Verification items for this drawing (mm, ordinates from the low corner). A direction names the side the tool comes from. Round coordinates to 2 decimals unless told otherwise and drop trailing zeros. Order: outer loops, then holes, each group sorted by start corner. A loop starts at its lowest first (then second) coordinate and runs counter-clockwise, first axis right, second up. Notation, with made-up numbers: (-8.75, -14.5) -> (8.25, -14.5) arc R19 ccw to (8.25, -2.5) -> close; hole circle Ø11 at (29, -28.75). An arc over 180 degrees is marked (long way). Answer in a Markdown table with one row per item. Add a question column.
1. Sectioned sample at B-B, the plane y = 33. Record the boundary of the cut face in (x, z) (3 decimals).
2. Access from +Z, -Z, +X, -X, +Y, -Y to the whole of each face (thin tool, end or side, straight path). Record for the marked faces 4 and 5.
3. Material ranges on L1, parallel to Z at x = 155, y = 62; L2, parallel to X at y = 96.5, z = 453, recorded low to high. Write a range as from..to.
4. Depth check by flat-ended pin: P1, Ø10, axis at x = 90, y = 67.5, coming from the -Z side; P2, Ø10, axis at y = 71, z = 347.5, coming from the +X side. Enter the tip coordinate at first touch or a pass-through.
5. Draft check along Z on the marked faces 1, 2 and 3. Enter one of: +Z half, -Z half, draft (parallel to the pull), parting line (faces both ways), or undercut.
6. Sectioned sample at C-C, the plane z = 95.5. Record the boundary of the cut face in (x, y).
7. Sectioned sample at A-A, the plane x = 233. Record the boundary of the cut face in (y, z), then the cut area to 3 significant figures.
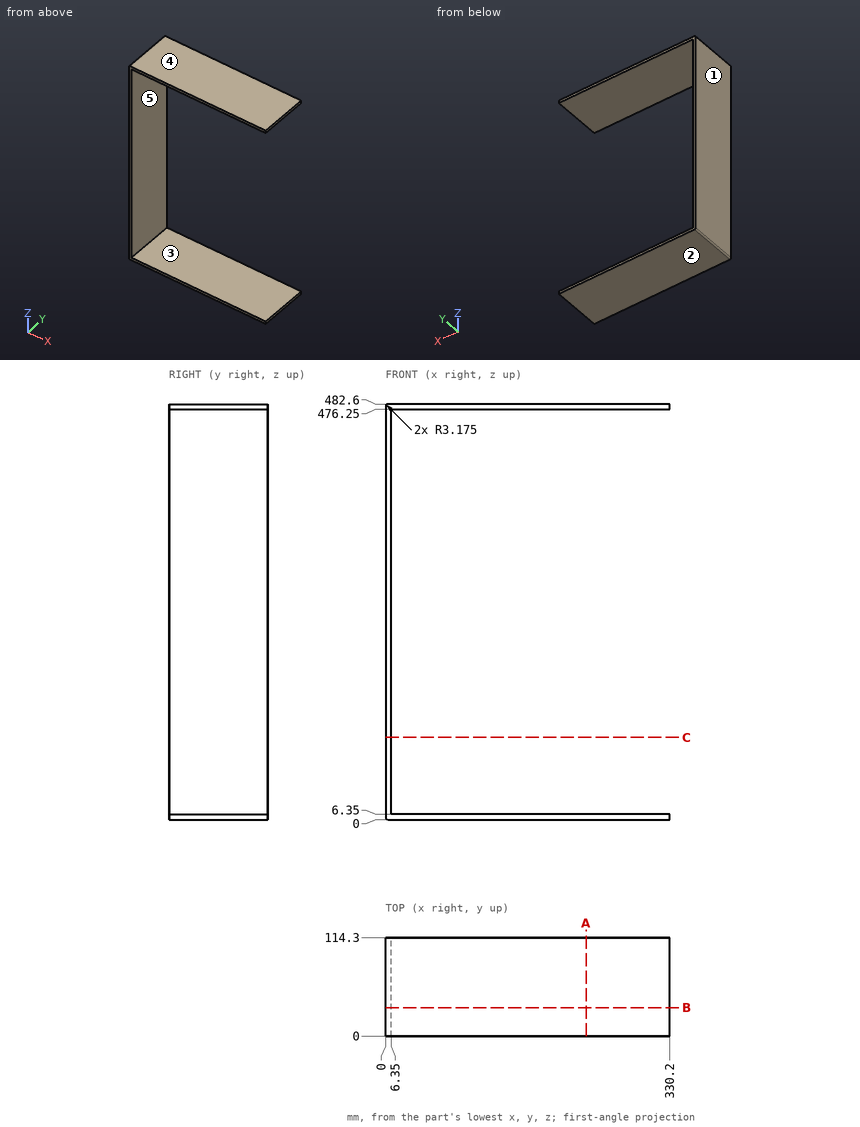
Answer key:
| question | item | result |
|---|---|---|
| 1 | outline | (0, 3.175) arc R3.175 ccw to (3.175, 0) -> (330.2, 0) -> (330.2, 6.35) -> (6.35, 6.35) -> (6.35, 476.25) -> (330.2, 476.25) -> (330.2, 482.6) -> (3.175, 482.6) arc R3.175 ccw to (0, 479.425) -> close |
| 2 | face 4 | +Z, +X, -X, +Y, -Y |
| 2 | face 5 | +X, +Y, -Y |
| 3 | L1 | z = 0..6.35, 476.25..482.6 |
| 3 | L2 | x = 0..6.35 |
| 4 | P1 | stops at z = 0 |
| 4 | P2 | stops at x = 6.35 |
| 5 | face 1 | draft |
| 5 | face 2 | -Z half |
| 5 | face 3 | undercut |
| 6 | outline | (0, 0) -> (6.35, 0) -> (6.35, 114.3) -> (0, 114.3) -> close |
| 7 | outline | (0, 0) -> (114.3, 0) -> (114.3, 6.35) -> (0, 6.35) -> close; (0, 476.25) -> (114.3, 476.25) -> (114.3, 482.6) -> (0, 482.6) -> close |
| 7 | area | 1,450 mm² |
